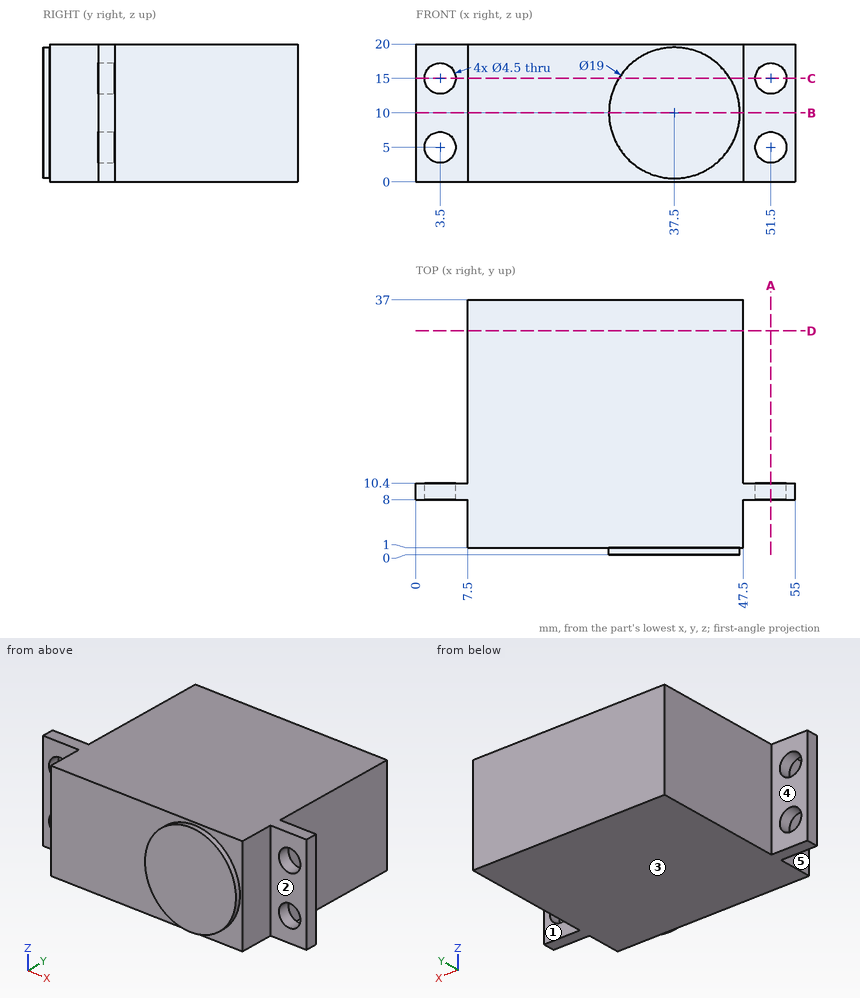
Geometry check sheet. Reference: drawing and pictorial views, mm from the part's lowest x, y, z. A direction names the side the tool comes from. Coordinates: 2 decimals unless noted, no trailing zeros. Write each loop counter-clockwise with the first axis right and the second up, starting at its lowest first coordinate (ties: lowest second). Pieces come first, ordered by that corner, then holes. Notation, with made-up numbers: (69.5, 66) - (104.5, 66) arc R25 ccw to (104.5, 101) - close; hole circle Ø9 at (-11.5, -4.5). An arc over 180 degrees is marked (long way). One line per question, with ' | ' between items. Start each with the question number.
1. Section check C-C (z = 15). Enter the section's corners in (x, y).
2. Section check B-B (z = 10). Enter the section's corners in (x, y).
3. Material ranges on line 1 along Z through (x, y) = (3.5, 9.55); line 2 along Y through (x, z) = (14, 15); line 3 along Y through (x, z) = (50.5, 18.75), recorded low to high.
4. Section check A-A (x = 51.5). Enter the section's corners in (y, z), plus the area to 3 significant figures.
5. Access from +Z, -Z, +X, -X, +Y, -Y to the whole of each face (thin tool, end or side, straight path). Record for the marked faces 1, 2, 3, 4 and 5.
6. Gauge pin test, flat ends, axial feed: P1, Ø2, axis at x = 5, z = 11, coming from the -Y side; P2, Ø7, axis at x = 3.5, z = 5, coming from the +Y side; P3, Ø8, axis at y = 30, z = 10.5, coming from the +X side; P4, Ø4, axis at x = 51.5, z = 15, coming from the +Y side. Record the tip position at first contact, or that the pin passes through.
7. Section check D-D (y = 32.5). Enter the section's corners in (x, z).
Computed values:
1) outline: (0, 8) - (1.25, 8) - (1.25, 10.4) - (0, 10.4) - close; (5.75, 8) - (7.5, 8) - (7.5, 1) - (29.42, 1) - (29.42, 0) - (45.58, 0) - (45.58, 1) - (47.5, 1) - (47.5, 8) - (49.25, 8) - (49.25, 10.4) - (47.5, 10.4) - (47.5, 37) - (7.5, 37) - (7.5, 10.4) - (5.75, 10.4) - close; (53.75, 8) - (55, 8) - (55, 10.4) - (53.75, 10.4) - close
2) outline: (0, 8) - (7.5, 8) - (7.5, 1) - (28, 1) - (28, 0) - (47, 0) - (47, 1) - (47.5, 1) - (47.5, 8) - (55, 8) - (55, 10.4) - (47.5, 10.4) - (47.5, 37) - (7.5, 37) - (7.5, 10.4) - (0, 10.4) - close
3) line 1: 0 to 2.75, 7.25 to 12.75, 17.25 to 20 | line 2: 1 to 37 | line 3: 8 to 10.4
4) outline: (8, 0) - (10.4, 0) - (10.4, 2.75) - (8, 2.75) - close; (8, 7.25) - (10.4, 7.25) - (10.4, 12.75) - (8, 12.75) - close; (8, 17.25) - (10.4, 17.25) - (10.4, 20) - (8, 20) - close | area: 26.4 mm²
5) face 1: +Z, -Z, +X, +Y | face 2: +Z, -Z, +X, -Y | face 3: -Z, +X, -X, +Y, -Y | face 4: +Z, -Z, -X, +Y | face 5: +Z, -Z, -X, -Y
6) P1: y = 8 | P2: y = 10.4 | P3: x = 47.5 | P4: through
7) outline: (7.5, 0) - (47.5, 0) - (47.5, 20) - (7.5, 20) - close
